from build123d import *

# Parameters (mm, degrees)
SKETCH1_W           = 40.3
SKETCH1_H           = 20
BOSS_EXTRUDE1_DEPTH = 40.1
SKETCH2_W           = 20
SKETCH2_H           = 2.5
BOSS_EXTRUDE2_DEPTH = 7
SKETCH3_W           = 20
SKETCH3_H           = 2.5
BOSS_EXTRUDE3_DEPTH = 7
SKETCH4_R           = 1.5
CUT_EXTRUDE1_DEPTH  = 7
SKETCH5_R           = 3
BOSS_EXTRUDE4_DEPTH = 3.5


with BuildPart() as part:
    # Sketch1 → Boss-Extrude1 (new body)
    with BuildSketch(Plane(origin=(0, 0, 0), x_dir=(1, 0, 0), z_dir=(0, 1, 0))):
        Rectangle(SKETCH1_W, SKETCH1_H)
    extrude(amount=BOSS_EXTRUDE1_DEPTH)

    # Sketch2 → Boss-Extrude2 (add)
    with BuildSketch(Plane(origin=(20.15, 0, 0), x_dir=(0, 0, -1), z_dir=(1, 0, 0))):
        with Locations((0, 12.25)):
            Rectangle(SKETCH2_W, SKETCH2_H)
    extrude(amount=BOSS_EXTRUDE2_DEPTH)

    # Sketch3 → Boss-Extrude3 (add)
    with BuildSketch(Plane.ZY.offset(20.15)):
        with Locations((0, 12.25)):
            Rectangle(SKETCH3_W, SKETCH3_H)
    extrude(amount=BOSS_EXTRUDE3_DEPTH)

    # Sketch4 → Cut-Extrude1 (cut)
    with BuildSketch(Plane.XZ.offset(-11)):
        with Locations(Location((-24.15, 5, 0), (0, 0, 270))):
            Circle(SKETCH4_R)
        with Locations(Location((-24.15, -5, 0), (0, 0, 270))):
            Circle(SKETCH4_R)
        with Locations(Location((24.15, 5, 0), (0, 0, 270))):
            Circle(SKETCH4_R)
        with Locations(Location((24.15, -5, 0), (0, 0, 270))):
            Circle(SKETCH4_R)
    extrude(amount=-CUT_EXTRUDE1_DEPTH, mode=Mode.SUBTRACT)

    # Sketch5 → Boss-Extrude4 (add)
    with BuildSketch(Plane.XZ):
        with Locations(Location((11.15, 0, 0), (0, 0, 270))):
            Circle(SKETCH5_R)
    extrude(amount=BOSS_EXTRUDE4_DEPTH)


solid = part.part
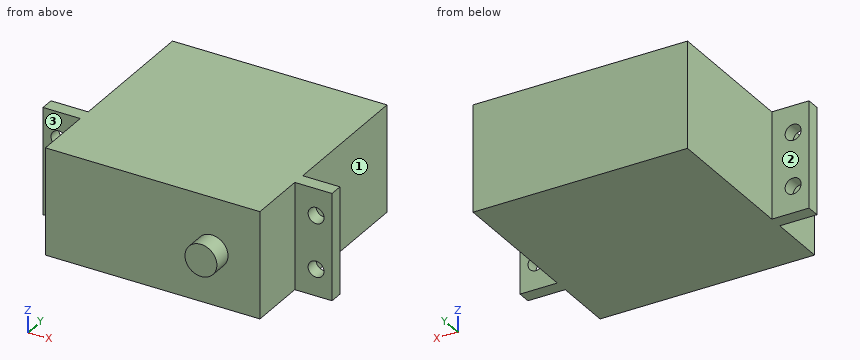
The listing builds one solid part. Answer for the finished solid, in the listing's coordinates (mm). Face numbers are marked on the shaded views. A direction names the side the tool comes from. Coordinates: 2 decimals unless noted, no trailing zeros. Write each loop counter-clockwise with the first axis right and the second up, starting at its lowest first coordinate (ties: lowest second). Pieces come first, ordered by that corner, then holes. Notation, with made-up numbers: (77.25, -13) - (116.25, -13) arc R16 cw to (116.25, -8) - close; hole circle Ø10 at (48.25, 24). An arc over 180 degrees is marked (long way). Return JSON: item names as keys, results as strings.
1. The part is cut by section C-C on x = 11.15. Determine the outline of the cut face in (y, z).
Final values:
{"outline": "(-3.5, -3) - (0, -3) - (0, -10) - (40.1, -10) - (40.1, 10) - (0, 10) - (0, 3) - (-3.5, 3) - close"}
2. The part is cut by section B-B on z = 5. Determine the outline of the cut face in (x, y).
Final values:
{"outline": "(-27.15, 11) - (-25.65, 11) - (-25.65, 13.5) - (-27.15, 13.5) - close; (-22.65, 11) - (-20.15, 11) - (-20.15, 0) - (20.15, 0) - (20.15, 11) - (22.65, 11) - (22.65, 13.5) - (20.15, 13.5) - (20.15, 40.1) - (-20.15, 40.1) - (-20.15, 13.5) - (-22.65, 13.5) - close; (25.65, 11) - (27.15, 11) - (27.15, 13.5) - (25.65, 13.5) - close"}
3. Each of these flat-tipped pins is pushed along its axis until it touches: pin 1 Ø5.5 at (y, z) = (6, -4.5) entering from +X; pin 2 Ø2 at (x, z) = (-10, -3.5) entering from -Y; pin 3 Ø10 at (y, z) = (9.5, -1) entering from -X; pin 4 Ø3.5 at (x, z) = (25, 2) entering from +Y. Where does it stop, or does it pass through?
Final values:
{"pin 1": "x = 20.15", "pin 2": "y = 0", "pin 3": "x = -27.15", "pin 4": "y = 13.5"}
4. The part is cut by section A-A on x = -24.15. Determine the outline of the cut face in (y, z).
Final values:
{"outline": "(11, -10) - (13.5, -10) - (13.5, -6.5) - (11, -6.5) - close; (11, -3.5) - (13.5, -3.5) - (13.5, 3.5) - (11, 3.5) - close; (11, 6.5) - (13.5, 6.5) - (13.5, 10) - (11, 10) - close"}
5. Consider line 1 along X through (y, z) = (12.65, -5); line 2 along X through (y, z) = (26.5, 7); line 3 along Y through (x, z) = (-16, 6). Determine where each line is inside the solid, lowest interval first.
Final values:
{"line 1": "-27.15 to -25.65, -22.65 to 22.65, 25.65 to 27.15", "line 2": "-20.15 to 20.15", "line 3": "0 to 40.1"}
6. The part is cut by section D-D on z = 0. Determine the outline of the cut face in (x, y), then the cut area to 3 significant figures.
Final values:
{"outline": "(-27.15, 11) - (-20.15, 11) - (-20.15, 0) - (8.15, 0) - (8.15, -3.5) - (14.15, -3.5) - (14.15, 0) - (20.15, 0) - (20.15, 11) - (27.15, 11) - (27.15, 13.5) - (20.15, 13.5) - (20.15, 40.1) - (-20.15, 40.1) - (-20.15, 13.5) - (-27.15, 13.5) - close", "area": "1,670 mm^2"}
7. Which of the six approach directions +Z, -Z, +X, -X, +Y, -Y give full straight-line access (tool end or side, diameter ignored) to the marked faces 1, 2 and 3?
Final values:
{"face 1": "+Z, -Z, +X, +Y", "face 2": "+Z, -Z, -X, +Y", "face 3": "+Z, -Z, -X, -Y"}
